Autodesk Inventor part; units mm, degrees
ref_plane "YZ Plane" through (0, 0, 0) normal (1, 0, 0) x (0, 1, 0)
ref_plane "XZ Plane" through (0, 0, 0) normal (0, 1, 0) x (-1, 0, 0)
ref_plane "XY Plane" through (0, 0, 0) normal (0, 0, 1) x (1, 0, 0)
sketch "Sketch1" plane through (0, 0, 0) normal (0, 0, 1) x (1, 0, 0)
  line L0 (-6, -5.5) -> (6, -5.5)
  line L1 (6, -5.5) -> (6, 5.5)
  line L2 (6, 5.5) -> (-6, 5.5)
  line L3 (-6, 5.5) -> (-6, -5.5)
  point P0 (0, 0)
  point P1 (-6, 0)
  point P2 (0, 5.5)
  dimension "d0" = 12
  dimension "d1" = 11
extrude "Extrusion1" add sketch "Sketch1" along normal blind 4.5
sketch "Sketch2" plane through (0, 0, 4.5) normal (0, 0, 1) x (1, 0, 0)
  line L0 (6, -5.5) -> (6, 5.5)
  line L1 (6, 5.5) -> (-6, 5.5)
  line L2 (-6, 5.5) -> (-6, -5.5)
  line L3 (-6, -5.5) -> (6, -5.5)
  line L4 (6, -5.5) -> (6, 5.5)
  line L5 (6, 7.2241) -> (2.625, 5.9957)
  line L6 (2.625, 5.9957) -> (2.625, 5.0043)
  line L7 (2.625, 5.0043) -> (6, 3.7759)
  line L8 (6, 2.5117) -> (2.625, 1.2833)
  line L9 (2.625, 1.2833) -> (2.625, 0.292)
  line L10 (2.625, 0.292) -> (6, -0.9364)
  arc A0 (3, 6.1322) -> (2.625, 5.5965) centre (3.195, 5.5965) ccw
  arc A1 (2.625, 5.4035) -> (3, 4.8678) centre (3.195, 5.4035) ccw
  line L11 (6, 5.5) -> (-6, 5.5)
  arc A2 (2.625, 0.6911) -> (3, 0.1555) centre (3.195, 0.6911) ccw
  arc A3 (3, 1.4198) -> (2.625, 0.8841) centre (3.195, 0.8841) ccw
  line L12 (6, 7.2241) -> (6, 3.7759)
  line L13 (0, 5.5) -> (0.4792, -5.5)
  line L14 (0, -5.5) -> (6, -5.5)
  line L15 (-6.1272, 6.6958) -> (-2.6582, 5.7655)
  line L16 (-2.6582, 5.7655) -> (-2.572, 4.778)
  line L17 (-2.572, 4.778) -> (-5.8274, 3.2607)
  arc A4 (-2.6235, 5.3679) -> (-3.0437, 5.8689) centre (-3.1913, 5.3183) ccw
  arc A5 (-2.9337, 4.6094) -> (-2.6067, 5.1756) centre (-3.1745, 5.126) ccw
  line L18 (-6.1272, 6.6958) -> (-5.8274, 3.2607)
  line L19 (-5.7174, 2.0012) -> (-2.2484, 1.071)
  line L20 (-2.2484, 1.071) -> (-2.1622, 0.0834)
  line L21 (-2.1622, 0.0834) -> (-5.4176, -1.4338)
  arc A6 (-2.5239, -0.0852) -> (-2.1969, 0.481) centre (-2.7647, 0.4315) ccw
  arc A7 (-2.2137, 0.6734) -> (-2.6339, 1.1744) centre (-2.7815, 0.6238) ccw
  point P0 (0, 0)
  point P1 (0, 0)
  point P2 (2.625, 5.5)
  point P3 (4.5, 4.3219)
  point P4 (4.5, 1.9657)
  point P5 (2.625, 5.5)
  point P6 (6, -0.9364)
  point P7 (-2.6151, 5.2717)
  point P8 (-4.3805, 3.9351)
  point P9 (-6, 5.2386)
  point P10 (0, 7.2759)
  point P11 (-4.1756, 1.5878)
  point P12 (0, 2.5636)
  point P13 (0, 6.0117)
  point P14 (4.5, -0.3905)
  dimension "d14" = 70
  dimension "d15" = 4.7124
  dimension "d16" = 0.57
  dimension "d17" = 3.375
  dimension "d18" = 1.5
  dimension "d19" = 2.3562
  dimension "d48" = 2.3562
sketch "Sketch3" plane through (6, -5.5, 0) normal (1, 0, 0) x (0, 0, -1)
  line L0 (-4.5, 0) -> (-4.5, 11)
  line L1 (-4.5, 11) -> (-4.5, 0)
  line L2 (-4.5, 4.5636) -> (0, 2.9257)
  line L3 (0, 5.5) -> (0, 11)
  line L4 (0, 11) -> (-4.5, 11)
  dimension "d31" = 20
sweep "Sweep1" cut profiles "Sketch2" path "Sketch3" path curves L2 contours L10 A2 L9 A3 L8 L0 | L7 A1 L6 L1 L0 | L6 A0 L5 L12 L1
pattern_linear "Rectangular Pattern2" count 8 spacing 4.7124 along (0, -1, 0) of "Sweep1"
mirror "Mirror2" about plane through (0, 0, 0) normal (0, 0, -1)
ref_plane "Work Plane3" through (4.5, 2.8745, 4.5) normal (1, 0, 0) x (0, 0, -1)
sketch "Sketch6" plane through (0, 0, 4.5) normal (0, 0, 1) x (1, 0, 0)
  arc A0 (3, -3.2926) -> (2.625, -3.8283) centre (3.195, -3.8283) ccw
  line L0 (3, -3.2926) -> (6, -2.2007)
  line L1 (6, -2.2007) -> (6, -0.9364)
  line L2 (6, -0.9364) -> (3, 0.1555)
  arc A1 (2.625, 0.6911) -> (3, 0.1555) centre (3.195, 0.6911) ccw
  line L3 (2.625, 0.6911) -> (2.625, 0.8841)
  arc A2 (3, 1.4198) -> (2.625, 0.8841) centre (3.195, 0.8841) ccw
  line L4 (3, 1.4198) -> (6, 2.5117)
  line L5 (6, 2.5117) -> (6, 3.7759)
  line L6 (6, 3.7759) -> (3, 4.8678)
  arc A3 (2.625, 5.4035) -> (3, 4.8678) centre (3.195, 5.4035) ccw
  line L7 (2.625, 5.4035) -> (2.625, 5.5)
  line L8 (2.625, 5.5) -> (-6, 5.5)
  line L9 (-6, 5.5) -> (-6, -5.5)
  line L10 (-6, -5.5) -> (5.5911, -5.5)
  line L11 (-6, 4.0633) -> (-3.1875, 5.087)
  line L12 (-3.1875, 5.087) -> (-3.1875, 5.913)
  line L13 (2.625, 5.5) -> (-6, 5.5)
  line L14 (-3.1875, 5.913) -> (-6, 6.9367)
  line L15 (-6, 6.9367) -> (-6, 5.5)
  arc A4 (-3.5, 4.9732) -> (-3.1875, 5.4196) centre (-3.6625, 5.4196) ccw
  arc A5 (-3.1875, 5.5804) -> (-3.5, 6.0268) centre (-3.6625, 5.5804) ccw
  arc A6 (-3.5, 1.0462) -> (-3.1875, 1.4926) centre (-3.6625, 1.4926) ccw
  line L16 (-3.1875, 1.16) -> (-3.1875, 1.9861)
  arc A7 (-3.1875, 1.6535) -> (-3.5, 2.0998) centre (-3.6625, 1.6535) ccw
  line L17 (-3.1875, 1.9861) -> (-6, 3.0097)
  line L18 (-6, 3.0097) -> (-6, 1.573)
  line L19 (-6, 0.1363) -> (-3.1875, 1.16)
  arc A8 (-3.5, -2.8808) -> (-3.1875, -2.4344) centre (-3.6625, -2.4344) ccw
  line L20 (-3.1875, -2.767) -> (-3.1875, -1.9409)
  arc A9 (-3.1875, -2.2735) -> (-3.5, -1.8272) centre (-3.6625, -2.2735) ccw
  line L21 (-3.1875, -1.9409) -> (-6, -0.9173)
  line L22 (-6, -0.9173) -> (-6, -2.354)
  line L23 (-6, -3.7907) -> (-3.1875, -2.767)
  arc A10 (-3.5, -6.8078) -> (-3.1875, -6.3614) centre (-3.6625, -6.3614) ccw
  line L24 (-3.1875, -6.694) -> (-3.1875, -5.8679)
  arc A11 (-3.1875, -6.2005) -> (-3.5, -5.7542) centre (-3.6625, -6.2005) ccw
  line L25 (-3.1875, -5.8679) -> (-6, -4.8443)
  line L26 (-6, -4.8443) -> (-6, -6.281)
  line L27 (-6, -7.7177) -> (-3.1875, -6.694)
  line L28 (5.5911, -5.5) -> (3, -4.5569)
  arc A12 (2.625, -4.0213) -> (3, -4.5569) centre (3.195, -4.0213) ccw
  line L29 (2.625, -4.0213) -> (2.625, -3.8283)
  point P0 (0, 0)
  point P1 (-4.75, 6.4817)
  point P2 (-4.75, 4.5183)
  point P3 (-3.1875, 5.5)
  point P4 (-3.1875, 1.573)
  point P5 (-4.75, 2.5548)
  point P6 (-4.75, 0.5913)
  point P7 (-3.1875, -2.354)
  point P8 (-4.75, -1.3722)
  point P9 (-4.75, -3.3357)
  point P10 (-3.1875, -6.281)
  point P11 (-4.75, -5.2992)
  point P12 (-4.75, -7.2627)
  point P13 (-5.2013, -4.5)
  dimension "d50" = 70
  dimension "d51" = 1.25
  dimension "d52" = 1.5625
  dimension "d53" = 1.9635
  dimension "d54" = 0.475
  dimension "d57" = 3.927
extrude "Extrusion4" cut sketch "Sketch6" against normal blind 10 contours L9 L21 A9 L20 A8 L23 | A8 L20 L23 | L9 L17 A7 L16 A6 L19 | L21 L20 A9 | L12 A4 L11 L9 L8
ref_plane "Work Plane4" through (-4.75, 3.0097, -4.5) normal (-1, 0, 0) x (0, 0, 1)
sketch "Sketch7" plane through (0, 0, 0) normal (0, 1, 0) x (-1, 0, 0)
  circle A0 centre (0, 0) radius 2.25
  dimension "d65" = 4.5
extrude "Extrusion5" cut sketch "Sketch7" along normal through all both and the other way through all
equation "\"d15\" = 3.14159 * d18"
equation "\"d16\" = 0.38 * d18"
equation "\"d17\" = 2.25 * d18"
equation "\"d54\" = 0.38 * d51"
equation "\"d57\" = 3.14159 * d51"
equation "\"d32\" = 20.5deg"
properties part number "rack_3DPrint"
CAD build for the part. Positions are in the model's coordinates, mm. A direction names the side the tool comes from. Round coordinates to 2 decimals unless told otherwise and drop trailing zeros. Write each loop counter-clockwise with the first axis right and the second up, starting at its lowest first coordinate (ties: lowest second). Pieces come first, ordered by that corner, then holes. Notation, with made-up numbers: (2, 80.5) -> (16, 80.5) arc R22 cw to (16, 110.5) -> close; hole circle Ø11 at (60, 25.5). An arc over 180 degrees is marked (long way). Answer in a Markdown table with one row per item. Add a question column.
Item 1: Drop flat-ended pins along their axis: pin 1 Ø2.5 at (x, z) = (0, 0) entering from -Y; pin 2 Ø1 at (x, z) = (-4, 3.5) entering from +Y; pin 3 Ø1.4 at (y, z) = (5, -2.5) entering from +X. Give the stop position or say it passes through.
Item 2: Drill centre lines: line 1 (X direction, y = -2.6, z = 0); line 2 (Z direction, x = 0, y = 2.7); line 3 (Y direction, x = -3.25, z = -4). Where is each one in solid material? Low to high. Write a range as from..to.
Item 3: Mould opens along Z. For faces 3 (the face through (3.94, -5.17, -3.76)), 4 (the face through (-4.8, 4.5, 0.1)) say: pulls with the +Z half, pulls with the -Z half, needs draft (parallel to the pull), parting line crosses it, or undercut.
Item 4: Saw through at B-B, the plane x = 1.5. Write the cut outline in (y, z), then the cut area to 3 significant figures.
Item 5: Saw through at A-A, the plane x = 0. Write the cut outline in (y, z), then the cut area to 3 significant figures.
Item 6: Which spindle directions (+Z, -Z, +X, -X, +Y, -Y) get a long thin tool onto all of the face, cutting with end or side? Do faces 1 (the face through (4.47, -1.21, 2.22)), 2 (the face through (-4.732, 2.548, 0.063)). Say none if no direction does.
Findings below:
| question | item | result |
|---|---|---|
| 1 | pin 1 | passes through |
| 1 | pin 2 | stops at y = 4.97 |
| 1 | pin 3 | stops at x = 3.75 |
| 2 | line 1 | x = -3.19..-2.25, 2.25..6 |
| 2 | line 2 | z = -4.5..-2.25, 2.25..4.5 |
| 2 | line 3 | y = -5.5..-2.79, -1.92..1.26, 1.89..5.18 |
| 3 | face 3 | undercut |
| 3 | face 4 | needs draft |
| 4 | outline | (-5.5, -4.5) -> (5.5, -4.5) -> (5.5, -1.68) -> (-5.5, -1.68) -> close; (-5.5, 1.68) -> (5.5, 1.68) -> (5.5, 4.5) -> (-5.5, 4.5) -> close |
| 4 | area | 62.1 mm^2 |
| 5 | outline | (-5.5, -4.5) -> (5.5, -4.5) -> (5.5, -2.25) -> (-5.5, -2.25) -> close; (-5.5, 2.25) -> (5.5, 2.25) -> (5.5, 4.5) -> (-5.5, 4.5) -> close |
| 5 | area | 49.5 mm^2 |
| 6 | face 1 | +X |
| 6 | face 2 | +Z, -Z, -X |
